CAD build for the part. Positions are in the model's coordinates, mm. Coordinates: 2 decimals unless noted, no trailing zeros. Write each loop counter-clockwise with the first axis right and the second up, starting at its lowest first coordinate (ties: lowest second). Pieces come first, ordered by that corner, then holes. Notation, with made-up numbers: M -2,36 L 13,36 A20 ccw 13,42 Z; hole C 27,81 d3. An arc over 180 degrees is marked long. Put each result on its own line as item: value. Start each with the question number.
```python
from build123d import *

# Parameters (mm, degrees)
BOSS_EXTRUDE1_DEPTH = 4
SKETCH2_R           = 2
CUT_EXTRUDE1_DEPTH  = 4
SKETCH4_R           = 30
SKETCH4_R_2         = 2
SKETCH4_R_3         = 60
CUT_EXTRUDE2_DEPTH  = 4
SKETCH5_R           = 4.5
CUT_EXTRUDE3_DEPTH  = 4
SKETCH6_R           = 2
CUT_EXTRUDE4_DEPTH  = 4


with BuildPart() as part:
    # Sketch1 → Boss-Extrude1 (new body)
    with BuildSketch(Plane(origin=(0, 0, 0), x_dir=(1, 0, 0), z_dir=(0, 1, 0))):
        with BuildLine():
            Line((-219, 50), (-219, -100))
            Line((-219, -100), (-261, -100))
            Line((-261, -100), (-261, -120))
            Line((-261, -120), (-150, -160))
            Line((-150, -160), (150, -160))
            Line((150, -160), (261, -120))
            Line((261, -120), (261, -100))
            Line((261, -100), (219, -100))
            Line((219, -100), (219, 50))
            Line((219, 50), (261, 50))
            Line((261, 50), (261, 160))
            Line((261, 160), (110, 331.658711753))
            ThreePointArc((110, 331.658711753), (0, 382.155640476), (-110, 331.658711753))
            Line((-110, 331.658711753), (-261, 160))
            Line((-261, 160), (-261, 50))
            Line((-261, 50), (-219, 50))
        make_face()
    extrude(amount=BOSS_EXTRUDE1_DEPTH)

    # Sketch2 → Cut-Extrude1 (cut)
    with BuildSketch(Plane(origin=(0, 4, 0), x_dir=(1, 0, 0), z_dir=(0, 1, 0))):
        with Locations(Location((-206.3, -25, 0), (0, 0, 270))):
            Circle(SKETCH2_R)
        with Locations(Location((-206.3, 5, 0), (0, 0, 270))):
            Circle(SKETCH2_R)
        with Locations(Location((-206.3, 35, 0), (0, 0, 270))):
            Circle(SKETCH2_R)
        with Locations(Location((-206.3, -55, 0), (0, 0, 270))):
            Circle(SKETCH2_R)
        with Locations(Location((-206.3, -85, 0), (0, 0, 270))):
            Circle(SKETCH2_R)
        with Locations(Location((206.3, -85, 0), (0, 0, 270))):
            Circle(SKETCH2_R)
        with Locations(Location((206.3, -55, 0), (0, 0, 270))):
            Circle(SKETCH2_R)
        with Locations(Location((206.3, -25, 0), (0, 0, 270))):
            Circle(SKETCH2_R)
        with Locations(Location((206.3, 5, 0), (0, 0, 270))):
            Circle(SKETCH2_R)
        with Locations(Location((206.3, 35, 0), (0, 0, 270))):
            Circle(SKETCH2_R)
    extrude(amount=-CUT_EXTRUDE1_DEPTH, mode=Mode.SUBTRACT)

    # Sketch4 → Cut-Extrude2 (cut)
    with BuildSketch(Plane(origin=(0, 4, 0), x_dir=(1, 0, 0), z_dir=(0, 1, 0))):
        with Locations(Location((0, -100, 0), (0, 0, 270))):
            Circle(SKETCH4_R)
        with Locations(Location((-120.208152802, 215.208152802, 0), (0, 0, 270))):
            Circle(SKETCH4_R_2)
        with Locations(Location((0, 95, 0), (0, 0, 270))):
            Circle(SKETCH4_R_3)
        with Locations(Location((120.208152802, 215.208152802, 0), (0, 0, 270))):
            Circle(SKETCH4_R_2)
        with Locations(Location((120.208152802, -25.208152802, 0), (0, 0, 270))):
            Circle(SKETCH4_R_2)
        with Locations(Location((-120.208152802, -25.208152802, 0), (0, 0, 270))):
            Circle(SKETCH4_R_2)
        with Locations(Location((-120.208152802, 95, 0), (0, 0, 270))):
            Circle(SKETCH4_R_2)
        with Locations(Location((-120.208152802, 135, 0), (0, 0, 270))):
            Circle(SKETCH4_R_2)
        with Locations(Location((-120.208152802, 175, 0), (0, 0, 270))):
            Circle(SKETCH4_R_2)
        with Locations(Location((-120.208152802, 55, 0), (0, 0, 270))):
            Circle(SKETCH4_R_2)
        with Locations(Location((-120.208152802, 15, 0), (0, 0, 270))):
            Circle(SKETCH4_R_2)
        with Locations(Location((120.208152802, 15, 0), (0, 0, 270))):
            Circle(SKETCH4_R_2)
        with Locations(Location((120.208152802, 55, 0), (0, 0, 270))):
            Circle(SKETCH4_R_2)
        with Locations(Location((120.208152802, 95, 0), (0, 0, 270))):
            Circle(SKETCH4_R_2)
        with Locations(Location((120.208152802, 135, 0), (0, 0, 270))):
            Circle(SKETCH4_R_2)
        with Locations(Location((120.208152802, 175, 0), (0, 0, 270))):
            Circle(SKETCH4_R_2)
        with Locations(Location((-80.208152802, 215.208152802, 0), (0, 0, 270))):
            Circle(SKETCH4_R_2)
        with Locations(Location((-80.208152802, -25.208152802, 0), (0, 0, 270))):
            Circle(SKETCH4_R_2)
        with Locations(Location((-40.208152802, 215.208152802, 0), (0, 0, 270))):
            Circle(SKETCH4_R_2)
        with Locations(Location((-40.208152802, -25.208152802, 0), (0, 0, 270))):
            Circle(SKETCH4_R_2)
        with Locations(Location((-0.208152802, 215.208152802, 0), (0, 0, 270))):
            Circle(SKETCH4_R_2)
        with Locations(Location((-0.208152802, -25.208152802, 0), (0, 0, 270))):
            Circle(SKETCH4_R_2)
        with Locations(Location((39.791847198, 215.208152802, 0), (0, 0, 270))):
            Circle(SKETCH4_R_2)
        with Locations(Location((39.791847198, -25.208152802, 0), (0, 0, 270))):
            Circle(SKETCH4_R_2)
        with Locations(Location((79.791847198, 215.208152802, 0), (0, 0, 270))):
            Circle(SKETCH4_R_2)
        with Locations(Location((79.791847198, -25.208152802, 0), (0, 0, 270))):
            Circle(SKETCH4_R_2)
    extrude(amount=-CUT_EXTRUDE2_DEPTH, mode=Mode.SUBTRACT)

    # Sketch5 → Cut-Extrude3 (cut)
    with BuildSketch(Plane(origin=(0, 4, 0), x_dir=(1, 0, 0), z_dir=(0, 1, 0))):
        with Locations(Location((-30, 172, 0), (0, 0, 270))):
            Circle(SKETCH5_R)
        with Locations(Location((30, 172, 0), (0, 0, 270))):
            Circle(SKETCH5_R)
        with Locations(Location((30, 258, 0), (0, 0, 270))):
            Circle(SKETCH5_R)
        with Locations(Location((-30, 258, 0), (0, 0, 270))):
            Circle(SKETCH5_R)
    extrude(amount=-CUT_EXTRUDE3_DEPTH, mode=Mode.SUBTRACT)

    # Sketch6 → Cut-Extrude4 (cut)
    with BuildSketch(Plane(origin=(0, 4, 0), x_dir=(1, 0, 0), z_dir=(0, 1, 0))):
        with Locations(Location((0, 318.958711753, 0), (0, 0, 270))):
            Circle(SKETCH6_R)
        with Locations(Location((30, 318.958711753, 0), (0, 0, 270))):
            Circle(SKETCH6_R)
        with Locations(Location((60, 318.958711753, 0), (0, 0, 270))):
            Circle(SKETCH6_R)
        with Locations(Location((90, 318.958711753, 0), (0, 0, 270))):
            Circle(SKETCH6_R)
        with Locations(Location((-30, 318.958711753, 0), (0, 0, 270))):
            Circle(SKETCH6_R)
        with Locations(Location((-60, 318.958711753, 0), (0, 0, 270))):
            Circle(SKETCH6_R)
        with Locations(Location((-90, 318.958711753, 0), (0, 0, 270))):
            Circle(SKETCH6_R)
        with Locations(Location((0, -147.3, 0), (0, 0, 270))):
            Circle(SKETCH6_R)
        with Locations(Location((30, -147.3, 0), (0, 0, 270))):
            Circle(SKETCH6_R)
        with Locations(Location((60, -147.3, 0), (0, 0, 270))):
            Circle(SKETCH6_R)
        with Locations(Location((90, -147.3, 0), (0, 0, 270))):
            Circle(SKETCH6_R)
        with Locations(Location((-30, -147.3, 0), (0, 0, 270))):
            Circle(SKETCH6_R)
        with Locations(Location((-60, -147.3, 0), (0, 0, 270))):
            Circle(SKETCH6_R)
        with Locations(Location((-90, -147.3, 0), (0, 0, 270))):
            Circle(SKETCH6_R)
    extrude(amount=-CUT_EXTRUDE4_DEPTH, mode=Mode.SUBTRACT)


solid = part.part
```
(1) Slice it at A-A, the plane z = -109.5. Write the cut outline in (x, y), then the cut area to 3 significant figures.
(2) Drop flat-ended pins along their axis: pin 1 (8 mm diameter, centred on x = 30, z = -172, fed in from +Y); pin 2 (1.5 mm diameter, centred on y = 0.5, z = 54, fed in from +X). Give the stop position or say it passes through.
(3) Slice it at B-B, the plane y = 2.45. State how many separate pieces and enclosed holes the cut face has, then the cut area to 3 significant figures.
(4) Drill centre lines: line 1 (X direction, y = 1.9, z = -15); line 2 (X direction, y = 3, z = 55); line 3 (X direction, y = 1, z = -136.5). Where is each one in solid material? Low to high. Write a range as [from, to].
(5) Slice it at C-C, the plane x = 177. Write the cut outline in (y, z).
(6) Two-plate mould, pull along Z, no slides. Class faces 1 (the face through (2.64, 2.03, -154.94)), 2 (the face through (54, 4, -55)), 3 (the face through (-206.28, 1.97, 139.72)): +Z half, -Z half, draft (parallel to the pull), parting line (faces both ways), or undercut.
(7) Slice it at D-D, the plane z = -304. Write the cut outline in (x, y), then the cut area to 3 significant figures.
Result set:
1. outline: M -261,0 L -58.22,0 L -58.22,4 L -261,4 Z; M 58.22,0 L 261,0 L 261,4 L 58.22,4 Z
1. area: 1,620 mm^2
2. pin 1: passes through
2. pin 2: stops at x = 219
3. separate pieces: 1
3. enclosed holes: 54
3. area: 206,000 mm^2
4. line 1: x = [-219, -122.21], [-118.21, 118.21], [122.21, 219]
4. line 2: x = [-219, -208.3], [-204.3, 204.3], [208.3, 219]
4. line 3: x = [-261, -121.53], [-118.89, -43.33], [43.33, 118.89], [121.53, 261]
5. outline: M 0,-255.49 L 4,-255.49 L 4,150.27 L 0,150.27 Z
6. face 1: undercut
6. face 2: draft
6. face 3: +Z half
7. outline: M -134.33,0 L 134.33,0 L 134.33,4 L -134.33,4 Z
7. area: 1,070 mm^2
